```python
from build123d import *

# Parameters (mm, degrees)
BOSS_EXTRUDE1_DEPTH = 25
SKETCH2_R           = 20
CUT_EXTRUDE1_DEPTH  = 51
SKETCH3_W           = 80
SKETCH3_H           = 80
CUT_EXTRUDE2_DEPTH  = 15
SKETCH4_W           = 60
SKETCH4_H           = 90
BOSS_EXTRUDE2_DEPTH = 70
SKETCH5_W           = 25
SKETCH5_H           = 15
CUT_EXTRUDE3_DEPTH  = 60


with BuildPart() as part:
    # Sketch1 → Boss-Extrude1 (new body, symmetric)
    with BuildSketch(Plane.XY):
        with BuildLine():
            Line((-60, 0), (0, 0))
            Line((0, 0), (0, 80))
            Line((0, 80), (-60, 80))
            ThreePointArc((-60, 80), (-88.284271217, 68.284271278), (-100, 40.000000086))
            ThreePointArc((-100, 40.000000086), (-88.284271278, 11.715728783), (-60, 0))
        make_face()
    extrude(amount=BOSS_EXTRUDE1_DEPTH, both=True)

    # Sketch2 → Cut-Extrude1 (cut, through all)
    with BuildSketch(Plane.XY.offset(25)):
        with Locations((-60, 40)):
            Circle(SKETCH2_R)
    extrude(amount=-CUT_EXTRUDE1_DEPTH, mode=Mode.SUBTRACT)

    # Sketch3 → Cut-Extrude2 (cut, symmetric)
    with BuildSketch(Plane.XY):
        with Locations((-60, 40)):
            Rectangle(SKETCH3_W, SKETCH3_H)
    extrude(amount=CUT_EXTRUDE2_DEPTH, both=True, mode=Mode.SUBTRACT)

    # Sketch4 → Boss-Extrude2 (add)
    with BuildSketch(Plane(origin=(0, 0, 0), x_dir=(0, 0, -1), z_dir=(1, 0, 0))):
        with Locations((0, 40)):
            Rectangle(SKETCH4_W, SKETCH4_H)
    extrude(amount=BOSS_EXTRUDE2_DEPTH)

    # Sketch5 → Cut-Extrude3 (cut)
    with BuildSketch(Plane(origin=(70, 0, 0), x_dir=(0, 0, -1), z_dir=(1, 0, 0))):
        with Locations((0, 77.5)):
            Rectangle(SKETCH5_W, SKETCH5_H)
    extrude(amount=-CUT_EXTRUDE3_DEPTH, mode=Mode.SUBTRACT)


solid = part.part
```
Geometry check sheet. Reference: the model listing, model coordinates, mm. A direction names the side the tool comes from. Coordinates: 2 decimals unless noted, no trailing zeros. Write each loop counter-clockwise with the first axis right and the second up, starting at its lowest first coordinate (ties: lowest second). Pieces come first, ordered by that corner, then holes. Notation, with made-up numbers: (2.25, -14.5) -> (22.25, -14.5) arc R20 cw to (22.25, 15.5) -> close; hole circle Ø11 at (73, -8.75). An arc over 180 degrees is marked (long way). Use CSV: the item, a comma, the result in double quotes. Start each with the question number.
Item 1: Set-up check for faces 1 (the flat face through (-34, 41, -15)), 2 (the flat face through (0, 44, 27)), 3 (the flat face through (-17, 0, 0)), 4 (the flat face through (40, 77, 12.5)), 5 (the flat face through (-39.6, 40.6, -25)): record each of +Z, -Z, +X, -X, +Y, -Y from which the full face is reachable in a straight line by a thin tool's end or side.
Item 2: Cross-section at B-B, the plane x = -22. Record the cut outline in (y, z).
Item 3: Cross-section at C-C, the plane y = 35. Record the cut outline in (x, z).
Item 4: Mould release check, pull along Z, two halves, no side actions. Record for faces 6 (the flat face through (-16, 80, 0)), 7 (the flat face through (-39.6, 40.6, 25)), 8 (the flat face through (-20, 39, 0)): released by +Z, released by -Z, zero draft, split by the parting line, or undercut.
Item 5: Cross-section at A-A, the plane z = -20. Record the cut outline in (x, y).
Item 6: Cross-section at D-D, the plane x = -42. Record the cut outline in (y, z).
Item 7: Depth check by flat-ended pin: pin 1 Ø1 at (x, z) = (-6.5, -10) entering from -Y; pin 2 Ø8 at (y, z) = (28.5, -7.5) entering from -X; pin 3 Ø12 at (x, y) = (-22.5, 31) entering from +Z. Enter the tip coordinate at first touch or a pass-through.
Item 8: Thickness scan on line 1 (Y direction, x = -60, z = 17); line 2 (Z direction, x = -84.5, y = 60); line 3 (Z direction, x = 13, y = 78). Record the ranges inside material, lowest first.
Answers:
1,face 1,"-X, +Y, -Y"
1,face 2,"-X"
1,face 3,"+Z, -Z, -X, -Y"
1,face 4,"+X, +Y"
1,face 5,"-Z, -X, +Y, -Y"
2,outline,"(0, -25) -> (80, -25) -> (80, -15) -> (0, -15) -> close; (0, 15) -> (80, 15) -> (80, 25) -> (0, 25) -> close"
3,outline,"(-99.69, -25) -> (-79.36, -25) -> (-79.36, -15) -> (-99.69, -15) -> close; (-99.69, 15) -> (-79.36, 15) -> (-79.36, 25) -> (-99.69, 25) -> close; (-40.64, -25) -> (0, -25) -> (0, -30) -> (70, -30) -> (70, 30) -> (0, 30) -> (0, 25) -> (-40.64, 25) -> (-40.64, 15) -> (-20, 15) -> (-20, -15) -> (-40.64, -15) -> close"
4,face 6,"zero draft"
4,face 7,"released by +Z"
4,face 8,"undercut"
5,outline,"(-60, 0) -> (0, 0) -> (0, -5) -> (70, -5) -> (70, 85) -> (0, 85) -> (0, 80) -> (-60, 80) arc R40 ccw to start; hole circle Ø40 at (-60, 40)"
6,outline,"(0, -25) -> (31.28, -25) -> (31.28, -15) -> (0, -15) -> close; (0, 15) -> (31.28, 15) -> (31.28, 25) -> (0, 25) -> close; (48.72, -25) -> (80, -25) -> (80, -15) -> (48.72, -15) -> close; (48.72, 15) -> (80, 15) -> (80, 25) -> (48.72, 25) -> close"
7,pin 1,"y = 0"
7,pin 2,"x = -20"
7,pin 3,"z = 25"
8,line 1,"0 to 20, 60 to 80"
8,line 2,"-25 to -15, 15 to 25"
8,line 3,"-30 to -12.5, 12.5 to 30"
